```python
from build123d import *

# Parameters (mm, degrees)
PAD_DEPTH       = 10
FILLET_R        = 4.9
FILLET001_R     = 4.9
FILLET002_R     = 4.9
FILLET003_R     = 4.9
SKETCH001_R     = 2.1
POCKET_DEPTH    = 11.501
SKETCH002_R     = 2.1
POCKET001_DEPTH = 11.501


with BuildPart() as part:
    # Sketch → Pad (new body)
    with BuildSketch(Plane.XY):
        with BuildLine():
            Line((0, 0), (0, 10))
            ThreePointArc((1.5, 11.5), (0.43934, 11.06066), (0, 10))
            Line((1.5, 11.5), (11.5, 11.5))
            Line((11.5, 11.5), (11.5, 10.5))
            Line((1.5, 10.5), (11.5, 10.5))
            ThreePointArc((1.5, 10.5), (1.146447, 10.353553), (1, 10))
            Line((1, 0), (1, 10))
            Line((0, 0), (1, 0))
        make_face()
    extrude(amount=PAD_DEPTH)

    # Fillet
    fillet_edges = [part.edges().sort_by_distance(p)[0] for p in [
        (0.5, 0, 10),
    ]]
    fillet(fillet_edges, radius=FILLET_R)

    # Fillet001
    fillet001_edges = [part.edges().sort_by_distance(p)[0] for p in [
        (0.5, 0, 0),
    ]]
    fillet(fillet001_edges, radius=FILLET001_R)

    # Fillet002
    fillet002_edges = [part.edges().sort_by_distance(p)[0] for p in [
        (11.5, 11, 0),
    ]]
    fillet(fillet002_edges, radius=FILLET002_R)

    # Fillet003
    fillet003_edges = [part.edges().sort_by_distance(p)[0] for p in [
        (11.5, 11, 10),
    ]]
    fillet(fillet003_edges, radius=FILLET003_R)

    # Sketch001 → Pocket (cut, through all)
    with BuildSketch(Plane(origin=(0, 0, 0), x_dir=(0, -1, 0), z_dir=(-1, 0, 0))):
        with Locations((-5, 5)):
            Circle(SKETCH001_R)
    extrude(amount=-POCKET_DEPTH, mode=Mode.SUBTRACT)

    # Sketch002 → Pocket001 (cut, through all)
    with BuildSketch(Plane(origin=(0, 11.5, 0), x_dir=(-1, 0, 0), z_dir=(0, 1, 0))):
        with Locations((-6.5, 5)):
            Circle(SKETCH002_R)
    extrude(amount=-POCKET001_DEPTH, mode=Mode.SUBTRACT)


solid = part.part
```
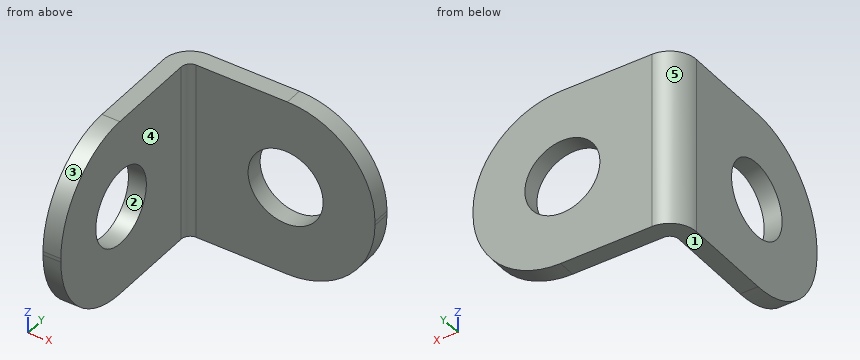
The listing builds one solid part. Answer for the finished solid, in the listing's coordinates (mm). Face numbers are marked on the shaded views. A direction names the side the tool comes from. Give positions to 0.01 mm unless a question says otherwise; leave off trailing zeros. Order: outer loops, then holes, each group sorted by start corner. A loop starts at its lowest first (then second) coordinate and runs counter-clockwise, first axis right, second up. Notation, with made-up numbers: (8.5, 45.25) -> (48.5, 45.25) arc R13 cw to (48.5, 52.25) -> close; hole circle Ø1 at (74, 43). An arc over 180 degrees is marked (long way). Write each question's results on one line, items separated by ' | '.
Q1. The part is cut by section A-A, the plane x = 5.5. Give the vertices of the cut face in (y, z), and give its area (3 significant figures).
Checked values:
outline: (10.5, 0) -> (11.5, 0) -> (11.5, 3.15) -> (10.5, 3.15) -> close; (10.5, 6.85) -> (11.5, 6.85) -> (11.5, 10) -> (10.5, 10) -> close | area: 6.31 mm^2
Q2. Determine the mould class of the marked faces 1, 2 and 3 for opening direction Z: pulls with the +Z half, pulls with the -Z half, needs draft (parallel to the pull), parting line crosses it, or undercut.
Checked values:
face 1: pulls with the -Z half | face 2: undercut | face 3: pulls with the +Z half
Q3. The part is cut by section C-C, the plane z = 6. Give the vertices of the cut face in (x, y), and give its area (3 significant figures).
Checked values:
outline: (0, 0.08) -> (1, 0.08) -> (1, 3.15) -> (0, 3.15) -> close; (0, 6.85) -> (1, 6.85) -> (1, 10) arc R0.5 cw to (1.5, 10.5) -> (4.65, 10.5) -> (4.65, 11.5) -> (1.5, 11.5) arc R1.5 ccw to (0, 10) -> close; (8.35, 10.5) -> (11.42, 10.5) -> (11.42, 11.5) -> (8.35, 11.5) -> close | area: 14.0 mm^2
Q4. Straight lines are drawn through the part: probe 1 along Z at (x, y) = (0.3, 5); probe 2 along X at (y, z) = (1.5, 5.5); probe 3 along Y at (x, z) = (11, 5.5). For each, find the intervals that lie inside material, in ascending order. Write a range as from..to.
Checked values:
probe 1: z = 0..2.9, 7.1..10 | probe 2: x = 0..1 | probe 3: y = 10.5..11.5
Q5. The part is cut by section D-D, the plane z = 7.5. Give the vertices of the cut face in (x, y).
Checked values:
outline: (0, 0.63) -> (1, 0.63) -> (1, 10) arc R0.5 cw to (1.5, 10.5) -> (10.87, 10.5) -> (10.87, 11.5) -> (1.5, 11.5) arc R1.5 ccw to (0, 10) -> close
Q6. Each of these flat-tipped pins is pushed along its axis until it touches: P1, Ø4, axis at x = 6.5, z = 5, coming from the -Y side; P2, Ø4, axis at x = 9.5, z = 8, coming from the -Y side. Where does it stop, or does it pass through?
Checked values:
P1: passes through | P2: stops at y = 10.5
Q7. Which of the six approach directions +Z, -Z, +X, -X, +Y, -Y give full straight-line access (tool end or side, diameter ignored) to the marked faces 4 and 5?
Checked values:
face 4: +Z, -Z, +X, -Y | face 5: +Z, -Z, -X, +Y
Q8. The part is cut by section B-B, the plane y = 4.25. Give the vertices of the cut face in (x, z), and give its area (3 significant figures).
Checked values:
outline: (0, 0.04) -> (1, 0.04) -> (1, 3.04) -> (0, 3.04) -> close; (0, 6.96) -> (1, 6.96) -> (1, 9.96) -> (0, 9.96) -> close | area: 5.99 mm^2
